```python
from build123d import *

# Parameters (mm, degrees)
SKETCH1_W                          = 2.5
SKETCH1_H                          = 4.25
CUT_EXTRUDE1_DEPTH                 = 7.509608283
CUT_EXTRUDE2_DEPTH                 = 7.509608283
CUT_EXTRUDE3_DEPTH                 = 7.509608283
CUT_EXTRUDE4_DEPTH                 = 7.509608283
CUT_EXTRUDE5_DEPTH                 = 7.509608283
CUT_EXTRUDE6_DEPTH                 = 7.509608283
CUT_EXTRUDE7_DEPTH                 = 7.509608283
CUT_EXTRUDE8_DEPTH                 = 7.509608283
CUT_EXTRUDE9_DEPTH                 = 7.509608283
CUT_EXTRUDE10_DEPTH                = 7.509608283
CUT_EXTRUDE11_DEPTH                = 7.500982013
CUT_EXTRUDE12_DEPTH                = 7.500982013
CUT_EXTRUDE13_DEPTH                = 7.500982013
CUT_EXTRUDE14_DEPTH                = 7.500982013
CUT_EXTRUDE15_DEPTH                = 7.500982013
SKETCH17_W                         = 3.8000508
SKETCH17_H                         = 3
F_4_0_4_DIAMETER_HOLE1_D           = 4
BOSS_EXTRUDE2_DEPTH                = 6.3000508
TAP_DRILL_FOR_M2_5X0_45_TAP1_D     = 2.05
TAP_DRILL_FOR_M2_5X0_45_TAP1_DEPTH = 3


with BuildPart() as part:
    # Sketch1 → Revolve1 (revolve)
    with BuildSketch(Plane(origin=(0, 0, 0), x_dir=(-1, 0, 0), z_dir=(0, 0, -1)), mode=Mode.PRIVATE) as revolve1_sk:
        with Locations((-1.25, 2.125)):
            Rectangle(SKETCH1_W, SKETCH1_H)
    revolve(revolve1_sk.sketch.rotate(Axis((2.5, 0, 0), (-1, 0, 0)), 270), axis=Axis((2.5, 0, 0), (-1, 0, 0)))

    # Sketch2 → Cut-Extrude1 (cut, through all)
    with BuildSketch(Plane(origin=(2.5, 0, 0), x_dir=(0, 0, -1), z_dir=(1, 0, 0))):
        with BuildLine():
            ThreePointArc((2.585993953, 3.372704445), (2.472774023, 2.780247912), (2.135335156, 2.280289405))
            ThreePointArc((2.135335156, 2.280289405), (2.321584435, 2.090364014), (2.491001044, 1.88528242))
            ThreePointArc((2.491001044, 1.88528242), (3.023492692, 2.168612866), (3.624538392, 2.219283994))
            ThreePointArc((3.624538392, 2.219283994), (3.158365508, 2.843805077), (2.585993953, 3.372704445))
        make_face()
    extrude(amount=-CUT_EXTRUDE1_DEPTH, mode=Mode.SUBTRACT)

    # Sketch3 → Cut-Extrude2 (cut, through all)
    with BuildSketch(Plane(origin=(2.5, 0, 0), x_dir=(0, 0, -1), z_dir=(1, 0, 0))):
        with BuildLine():
            ThreePointArc((3.734225512, 2.029300328), (3.389820178, 1.534115047), (2.87820299, 1.214628975))
            ThreePointArc((2.87820299, 1.214628975), (2.971100557, 0.96536909), (3.042456131, 0.709109787))
            ThreePointArc((3.042456131, 0.709109787), (3.644152332, 0.751361165), (4.213844705, 0.553184234))
            ThreePointArc((4.213844705, 0.553184234), (4.041990194, 1.313322226), (3.734225512, 2.029300328))
        make_face()
    extrude(amount=-CUT_EXTRUDE2_DEPTH, mode=Mode.SUBTRACT)

    # Sketch4 → Cut-Extrude3 (cut, through all)
    with BuildSketch(Plane(origin=(2.5, 0, 0), x_dir=(0, 0, -1), z_dir=(1, 0, 0))):
        with BuildLine():
            ThreePointArc((4.236775558, 0.335011746), (3.72073563, 0.022719752), (3.12340338, -0.061051839))
            ThreePointArc((3.12340338, -0.061051839), (3.106886401, -0.326546919), (3.067842913, -0.589674367))
            ThreePointArc((3.067842913, -0.589674367), (3.634704928, -0.795807707), (4.074538988, -1.208566106))
            ThreePointArc((4.074538988, -1.208566106), (4.226718055, -0.444245969), (4.236775558, 0.335011746))
        make_face()
    extrude(amount=-CUT_EXTRUDE3_DEPTH, mode=Mode.SUBTRACT)

    # Sketch5 → Cut-Extrude4 (cut, through all)
    with BuildSketch(Plane(origin=(2.5, 0, 0), x_dir=(0, 0, -1), z_dir=(1, 0, 0))):
        with BuildLine():
            ThreePointArc((4.00674862, -1.417203408), (3.40830209, -1.492603993), (2.82853895, -1.326176235))
            ThreePointArc((2.82853895, -1.326176235), (2.705463361, -1.562), (2.562771785, -1.786498468))
            ThreePointArc((2.562771785, -1.786498468), (2.996784021, -2.205374197), (3.230708464, -2.761344386))
            ThreePointArc((3.230708464, -2.761344386), (3.680607966, -2.124999999), (4.00674862, -1.417203408))
        make_face()
    extrude(amount=-CUT_EXTRUDE4_DEPTH, mode=Mode.SUBTRACT)

    # Sketch6 → Cut-Extrude5 (cut, through all)
    with BuildSketch(Plane(origin=(2.5, 0, 0), x_dir=(0, 0, -1), z_dir=(1, 0, 0))):
        with BuildLine():
            ThreePointArc((3.083918444, -2.92437122), (2.506542154, -2.749842949), (2.044594439, -2.361992714))
            ThreePointArc((2.044594439, -2.361992714), (1.836241128, -2.52736909), (1.614574134, -2.674420753))
            ThreePointArc((1.614574134, -2.674420753), (1.840691933, -3.233611452), (1.828259097, -3.836661137))
            ThreePointArc((1.828259097, -3.836661137), (2.498087322, -3.438322226), (3.083918444, -2.92437122))
        make_face()
    extrude(amount=-CUT_EXTRUDE5_DEPTH, mode=Mode.SUBTRACT)

    # Sketch7 → Cut-Extrude6 (cut, through all)
    with BuildSketch(Plane(origin=(2.5, 0, 0), x_dir=(0, 0, -1), z_dir=(1, 0, 0))):
        with BuildLine():
            ThreePointArc((1.627850754, -3.925888679), (1.17137831, -3.531609077), (0.907120976, -2.989399193))
            ThreePointArc((0.907120976, -2.989399193), (0.649516122, -3.055733105), (0.387201946, -3.099911394))
            ThreePointArc((0.387201946, -3.099911394), (0.366327487, -3.702727912), (0.109687121, -4.248584321))
            ThreePointArc((0.109687121, -4.248584321), (0.883624686, -4.157127303), (1.627850754, -3.925888679))
        make_face()
    extrude(amount=-CUT_EXTRUDE6_DEPTH, mode=Mode.SUBTRACT)

    # Sketch8 → Cut-Extrude7 (cut, through all)
    with BuildSketch(Plane(origin=(2.5, 0, 0), x_dir=(0, 0, -1), z_dir=(1, 0, 0))):
        with BuildLine():
            ThreePointArc((-0.109687122, -4.248584322), (-0.366327487, -3.702727912), (-0.387201947, -3.099911394))
            ThreePointArc((-0.387201947, -3.099911394), (-0.649516122, -3.055733105), (-0.907120975, -2.989399193))
            ThreePointArc((-0.907120975, -2.989399193), (-1.171378309, -3.531609077), (-1.627850753, -3.92588868))
            ThreePointArc((-1.627850753, -3.92588868), (-0.883624686, -4.157127304), (-0.109687122, -4.248584322))
        make_face()
    extrude(amount=-CUT_EXTRUDE7_DEPTH, mode=Mode.SUBTRACT)

    # Sketch9 → Cut-Extrude8 (cut, through all)
    with BuildSketch(Plane(origin=(2.5, 0, 0), x_dir=(0, 0, -1), z_dir=(1, 0, 0))):
        with BuildLine():
            ThreePointArc((-1.828259096, -3.836661137), (-1.840691932, -3.233611453), (-1.614574133, -2.674420754))
            ThreePointArc((-1.614574133, -2.674420754), (-1.836241128, -2.527369091), (-2.044594439, -2.361992714))
            ThreePointArc((-2.044594439, -2.361992714), (-2.506542155, -2.749842949), (-3.083918444, -2.92437122))
            ThreePointArc((-3.083918444, -2.92437122), (-2.498087322, -3.438322226), (-1.828259096, -3.836661137))
        make_face()
    extrude(amount=-CUT_EXTRUDE8_DEPTH, mode=Mode.SUBTRACT)

    # Sketch10 → Cut-Extrude9 (cut, through all)
    with BuildSketch(Plane(origin=(2.5, 0, 0), x_dir=(0, 0, -1), z_dir=(1, 0, 0))):
        with BuildLine():
            ThreePointArc((-3.230708464, -2.761344387), (-2.996784021, -2.205374197), (-2.562771785, -1.786498468))
            ThreePointArc((-2.562771785, -1.786498468), (-2.705463361, -1.562), (-2.82853895, -1.326176236))
            ThreePointArc((-2.82853895, -1.326176236), (-3.40830209, -1.492603994), (-4.006748619, -1.417203409))
            ThreePointArc((-4.006748619, -1.417203409), (-3.680607966, -2.125), (-3.230708464, -2.761344387))
        make_face()
    extrude(amount=-CUT_EXTRUDE9_DEPTH, mode=Mode.SUBTRACT)

    # Sketch11 → Cut-Extrude10 (cut, through all)
    with BuildSketch(Plane(origin=(2.5, 0, 0), x_dir=(0, 0, -1), z_dir=(1, 0, 0))):
        with BuildLine():
            ThreePointArc((-4.074538989, -1.208566105), (-3.634704928, -0.795807707), (-3.067842914, -0.589674368))
            ThreePointArc((-3.067842914, -0.589674368), (-3.106886402, -0.326546919), (-3.12340338, -0.061051839))
            ThreePointArc((-3.12340338, -0.061051839), (-3.720735631, 0.022719752), (-4.236775558, 0.335011747))
            ThreePointArc((-4.236775558, 0.335011747), (-4.226718056, -0.444245968), (-4.074538989, -1.208566105))
        make_face()
    extrude(amount=-CUT_EXTRUDE10_DEPTH, mode=Mode.SUBTRACT)

    # Sketch12 → Cut-Extrude11 (cut, through all)
    with BuildSketch(Plane(origin=(2.5, 0, 0), x_dir=(0, 0, -1), z_dir=(1, 0, 0))):
        with BuildLine():
            ThreePointArc((-4.213844706, 0.553184234), (-3.644152332, 0.751361165), (-3.042456131, 0.709109788))
            ThreePointArc((-3.042456131, 0.709109788), (-2.971100557, 0.96536909), (-2.87820299, 1.214628975))
            ThreePointArc((-2.87820299, 1.214628975), (-3.389820179, 1.534115046), (-3.734225513, 2.029300326))
            ThreePointArc((-3.734225513, 2.029300326), (-4.041990195, 1.313322226), (-4.213844706, 0.553184234))
        make_face()
    extrude(amount=-CUT_EXTRUDE11_DEPTH, mode=Mode.SUBTRACT)

    # Sketch13 → Cut-Extrude12 (cut, through all)
    with BuildSketch(Plane(origin=(2.5, 0, 0), x_dir=(0, 0, -1), z_dir=(1, 0, 0))):
        with BuildLine():
            ThreePointArc((-2.585993952, 3.372704446), (-3.158365508, 2.843805077), (-3.624538391, 2.219283994))
            ThreePointArc((-3.624538391, 2.219283994), (-3.023492692, 2.168612865), (-2.491001044, 1.885282419))
            ThreePointArc((-2.491001044, 1.885282419), (-2.321584435, 2.090364014), (-2.135335156, 2.280289405))
            ThreePointArc((-2.135335156, 2.280289405), (-2.472774022, 2.780247912), (-2.585993952, 3.372704446))
        make_face()
    extrude(amount=-CUT_EXTRUDE12_DEPTH, mode=Mode.SUBTRACT)

    # Sketch14 → Cut-Extrude13 (cut, through all)
    with BuildSketch(Plane(origin=(2.5, 0, 0), x_dir=(0, 0, -1), z_dir=(1, 0, 0))):
        with BuildLine():
            ThreePointArc((-0.990620545, 4.132937326), (-1.728630733, 3.882568195), (-2.408516462, 3.501649391))
            ThreePointArc((-2.408516462, 3.501649391), (-1.880043697, 3.210891701), (-1.508829246, 2.735472593))
            ThreePointArc((-1.508829246, 2.735472593), (-1.270645273, 2.85391601), (-1.023248474, 2.951667081))
            ThreePointArc((-1.023248474, 2.951667081), (-1.128162774, 3.545650656), (-0.990620545, 4.132937326))
        make_face()
    extrude(amount=-CUT_EXTRUDE13_DEPTH, mode=Mode.SUBTRACT)

    # Sketch15 → Cut-Extrude14 (cut, through all)
    with BuildSketch(Plane(origin=(2.5, 0, 0), x_dir=(0, 0, -1), z_dir=(1, 0, 0))):
        with BuildLine():
            ThreePointArc((-0.776040155, 4.178547795), (-0.411518069, 3.69797819), (-0.265767165, 3.112674704))
            ThreePointArc((-0.265767165, 3.112674704), (0, 3.124), (0.265767165, 3.112674704))
            ThreePointArc((0.265767165, 3.112674704), (0.411518069, 3.69797819), (0.776040156, 4.178547795))
            ThreePointArc((0.776040156, 4.178547795), (0, 4.25), (-0.776040155, 4.178547795))
        make_face()
    extrude(amount=-CUT_EXTRUDE14_DEPTH, mode=Mode.SUBTRACT)

    # Sketch16 → Cut-Extrude15 (cut, through all)
    with BuildSketch(Plane(origin=(2.5, 0, 0), x_dir=(0, 0, -1), z_dir=(1, 0, 0))):
        with BuildLine():
            ThreePointArc((0.990620545, 4.132937326), (1.128162774, 3.545650656), (1.023248474, 2.951667081))
            ThreePointArc((1.023248474, 2.951667081), (1.270645273, 2.85391601), (1.508829246, 2.735472593))
            ThreePointArc((1.508829246, 2.735472593), (1.880043697, 3.210891701), (2.408516462, 3.50164939))
            ThreePointArc((2.408516462, 3.50164939), (1.728630733, 3.882568195), (0.990620545, 4.132937326))
        make_face()
    extrude(amount=-CUT_EXTRUDE15_DEPTH, mode=Mode.SUBTRACT)

    # Sketch17 → Revolve2 (revolve)
    with BuildSketch(Plane.XY, mode=Mode.PRIVATE) as revolve2_sk:
        with Locations((-1.9000254, 1.5)):
            Rectangle(SKETCH17_W, SKETCH17_H)
    revolve(revolve2_sk.sketch.rotate(Axis((-3.8000508, 0, 0), (1, 0, 0)), 270), axis=Axis((-3.8000508, 0, 0), (1, 0, 0)))

    # Ø4.0 (4) Diameter Hole1 (through all)
    with Locations(Plane(origin=(2.5, 0, 0), x_dir=(0, 0, -1), z_dir=(1, 0, 0))):
        with Locations((0, 0)):
            Hole(F_4_0_4_DIAMETER_HOLE1_D / 2)

    # Sketch21 → Boss-Extrude2 (add)
    with BuildSketch(Plane.ZY.offset(3.8000508)):
        with BuildLine():
            Line((-1.732050808, 1), (1.732050808, 1))
            ThreePointArc((1.732050808, 1), (0, 2), (-1.732050808, 1))
        make_face()
    extrude(amount=-BOSS_EXTRUDE2_DEPTH)

    # Tap Drill for M2.5x0.45 Tap1
    with Locations(Plane(origin=(-1.9000508, 2.999970615, 0.013278053), x_dir=(0, -0.004426017667, 0.999990205136), z_dir=(0, 0.999990205136, 0.004426017667))):
        with Locations((0, 0)):
            Hole(TAP_DRILL_FOR_M2_5X0_45_TAP1_D / 2, depth=TAP_DRILL_FOR_M2_5X0_45_TAP1_DEPTH)


solid = part.part
```
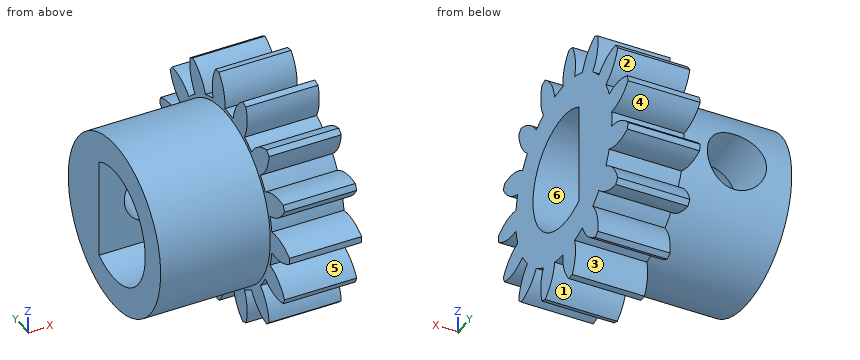
CAD build for the part. Positions are in the model's coordinates, mm. Face numbers are marked on the shaded views. A direction names the side the tool comes from. Coordinates: 2 decimals unless noted, no trailing zeros. Order: outer loops, then holes, each group sorted by start corner. A loop starts at its lowest first (then second) coordinate and runs counter-clockwise, first axis right, second up. Notation, with made-up numbers: (-9.75, 4) - (15.25, 4) arc R18 cw to (15.25, 37) - close; hole circle Ø3 at (5.5, 72.25). An arc over 180 degrees is marked (long way). Answer in a Markdown table with one row per item.
1. Slice it at B-B, the plane z = 0. Give the number of separate pieces and of enclosed holes in the cut face, then the cut area to 3 significant figures.
Answer:
| item | result |
|---|---|
| separate pieces | 3 |
| enclosed holes | 0 |
| area | 18.2 mm² |
2. Pull direction Y, two halves, no side cores. Call the marked faces 4, 5 and 6: +Y half, -Y half, draft (parallel to the pull), parting line (faces both ways), or undercut.
Answer:
| item | result |
|---|---|
| face 4 | +Y half |
| face 5 | -Y half |
| face 6 | undercut |
3. Flat gauge pins, fed straight in: P1, Ø1, axis at x = -1, y = 1.5, coming from the -Z side; P2, Ø1.5, axis at x = -1.5, y = 2.5, coming from the +Z side; P3, Ø2, axis at x = 0.5, y = -1, coming from the -Z side. Where does each tip first touch, or does it go through?
Answer:
| item | result |
|---|---|
| P1 | z = -2.83 |
| P2 | z = 2.44 |
| P3 | z = -4.07 |
4. Drill centre lines: L1, parallel to Z at x = -1, y = -1; L2, parallel to X at y = -1.75, z = -2.5; L3, parallel to Y at x = -0.75, z = 0. Where is each one in solid material? Low to high. Write a range as from..to.
Answer:
| item | result |
|---|---|
| L1 | -2.83..-1.73, 1.73..2.83 |
| L2 | 0..2.5 |
| L3 | -3..-2, 1..3 |
5. Slice it at C-C, the plane x = -1. List the corners of the cut face in (y, z).
Answer:
| item | result |
|---|---|
| outline | (1, -1.73) arc R2 cw (long way) to (1, 1.73) - (1, 0.49) - (2.96, 0.5) arc R3 ccw (long way) to (2.96, -0.48) - (1, -0.49) - close |
6. 3-axis set-ups, long thin cutter, end or side, ignore diameter. For the marked faces 1, 2 and 3: which of +Z, -Z, +X, -X, +Y, -Y reach the whole face in a straight line?
Answer:
| item | result |
|---|---|
| face 1 | -Z, +X, -X |
| face 2 | +X, -X, +Y |
| face 3 | +X, -X |
7. Slice it at A-A, the plane x = -0.25. List the corners of the cut face in (y, z).
Answer:
| item | result |
|---|---|
| outline | circle Ø6 at (0, 0); hole (1, -1.73) - (1, 1.73) arc R2 ccw (long way) to start |
